Autodesk Inventor part; units mm, degrees
ref_plane "YZ Plane" through (0, 0, 0) normal (1, 0, 0) x (0, 1, 0)
ref_plane "XZ Plane" through (0, 0, 0) normal (0, 1, 0) x (-1, 0, 0)
ref_plane "XY Plane" through (0, 0, 0) normal (0, 0, 1) x (1, 0, 0)
sketch "Sketch1" plane through (0, 0, 0) normal (0, 1, 0) x (-1, 0, 0)
  circle A0 centre (0, 0) radius 3
  dimension "d0" = 6
extrude "Extrusion1" add sketch "Sketch1" along normal blind 6
sketch "Sketch2" plane through (0, 6, 0) normal (0, 1, 0) x (1, 0, 0)
  circle A0 centre (0, 0) radius 3
  circle A1 centre (0, 0) radius 12
  dimension "d3" = 24
extrude "Extrusion2" add sketch "Sketch2" along normal blind 1 contours A0 | A1
sketch "Sketch3" plane through (0, 7, 0) normal (0, 1, 0) x (1, 0, 0)
  circle A0 centre (0, 0) radius 12
  line L0 (0, 0) -> (0, -9.5)
  line L1 (0, -9.5) -> (0, 9.5)
  circle A1 centre (0, -9.5) radius 1.5
  circle A2 centre (0, 9.5) radius 1.5
  dimension "d6" = 9.5
  dimension "d7" = 19
  dimension "d8" = 3
  dimension "d9" = 3
extrude "Extrusion3" add sketch "Sketch3" along normal blind 2 and the other way blind 3 contours A1 | A2
sketch "Sketch4" plane through (0, 0, 0) normal (0, -1, 0) x (1, 0, 0)
  circle A0 centre (0, 0) radius 3
extrude "Extrusion4" add sketch "Sketch4" along normal blind 2
properties part number "EE Wheel"
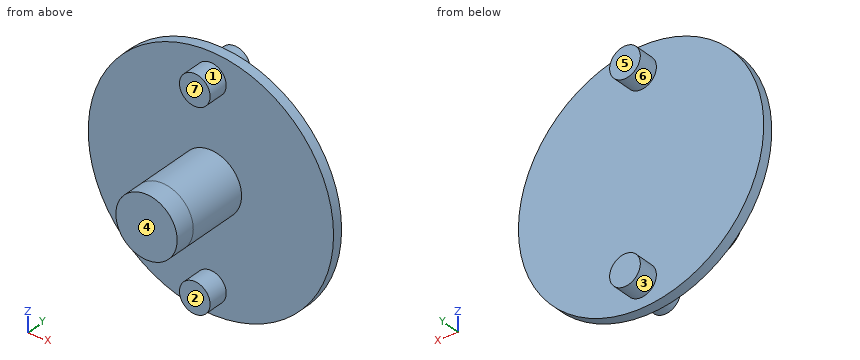
Can you work these out from the model? Positions are in its coordinate system, mm. Face numbers are marked on the shaded views. A direction names the side the tool comes from. Give positions to 0.01 mm unless a question says otherwise; leave off trailing zeros. Write each loop counter-clockwise with the first axis right and the second up, starting at its lowest first coordinate (ties: lowest second). Pieces come first, ordered by that corner, then holes. Notation, with made-up numbers: (-28, -27.5) -> (-17, -27.5) arc R15 cw to (-17, -16.5) -> close; hole circle Ø6 at (0, 1.25). An arc over 180 degrees is marked (long way). One line per item, written item: value.
Q1. Imagine slicing it at A-A on z = 0. Please give me the cut outline in (x, y).
Results found:
outline: (-12, 6) -> (-3, 6) -> (-3, -2) -> (3, -2) -> (3, 6) -> (12, 6) -> (12, 7) -> (-12, 7) -> close
Q2. Imagine slicing it at D-D on y = -1.5. Please give me the cut outline in (x, z), and give its area (3 significant figures).
Results found:
outline: circle Ø6 at (0, 0)
area: 28.3 mm^2
Q3. For P1, Ø3, axis at x = -4.5, y = 6, coming from the -Z side; P2, Ø0.9, axis at x = 0, z = 9.5, coming from the -Y side; P3, Ø12, axis at x = 0.5, z = -1.5, coming from the +Y side, each with a flat end and sliding along its axis, tell me the tip position at first contact or that it passes through.
Results found:
P1: stops at z = -11.62
P2: stops at y = 4
P3: stops at y = 7
Q4. Imagine slicing it at B-B on x = 0. Please give me the cut outline in (y, z).
Results found:
outline: (-2, -3) -> (6, -3) -> (6, -8) -> (4, -8) -> (4, -11) -> (6, -11) -> (6, -12) -> (7, -12) -> (7, -11) -> (9, -11) -> (9, -8) -> (7, -8) -> (7, 8) -> (9, 8) -> (9, 11) -> (7, 11) -> (7, 12) -> (6, 12) -> (6, 11) -> (4, 11) -> (4, 8) -> (6, 8) -> (6, 3) -> (-2, 3) -> close
Q5. Please list where these lines run through material, in increasing order: line 1 (Y direction, x = 3.75, z = 8.5); line 2 (Z direction, x = -0.75, y = 2); line 3 (Z direction, x = 2.25, y = 1.5). Write a range as [from, to].
Results found:
line 1: y = [6, 7]
line 2: z = [-2.9, 2.9]
line 3: z = [-1.98, 1.98]
Q6. Imagine slicing it at C-C on y = 4.75. Please give me the cut outline in (x, z), and give its area (3 significant figures).
Results found:
outline: circle Ø6 at (0, 0); circle Ø3 at (0, -9.5); circle Ø3 at (0, 9.5)
area: 42.4 mm^2
Q7. Which directions (+Z, -Z, +X, -X, +Y, -Y) give clear straight access to the entire face, cutting with the end or side of a thin tool? Please do the marked faces 1, 2, 3, 4 and 5.
Results found:
face 1: -Y
face 2: -Z, +X, -X, -Y
face 3: +Y
face 4: +Z, -Z, +X, -X, -Y
face 5: +Z, -Z, +X, -X, +Y
Q8. We'd pull the mould along Z, two halves only. Please class the marked faces 6 and 7: +Z half, -Z half, draft (parallel to the pull), parting line (faces both ways), or undercut.
Results found:
face 6: undercut
face 7: draft
